The listing builds one solid part. Answer for the finished solid, in the listing's coordinates (mm). A direction names the side the tool comes from. Coordinates: 2 decimals unless noted, no trailing zeros. Loops run counter-clockwise (first coordinate to the right, second up) from the corner with the lowest first, then second, coordinate; pieces in that order, holes last. Notation, with made-up numbers: M 28,65.5 L 55,65.5 A27 ccw 55,87.5 Z; hole C 44,85 d8. An arc over 180 degrees is marked long. Answer as a JSON object with one key per item and string values. Group by question number.
1. A cutting plane is placed at B-B on z = -3. Give the vertices of the cut face in (x, y) (3 decimals).
2. A cutting plane is placed at C-C on x = -25.5. Give the vertices of the cut face in (y, z) (3 decimals).
3. A cutting plane is placed at A-A on y = -25.4. Give the vertices of the cut face in (x, z), and give its area (3 significant figures).
4. For faces 1 (the face through (-18.455, -42.037, -14.166)), 2 (the face through (-57.15, -20, -23)), determine the directions among +Z, -Z, +X, -X, +Y, -Y from which every point of the face is accessible in a straight line to the end or side of a thin tool.
5. Determine the mould class of faces 3 (the face through (-29, 0, -16)), 4 (the face through (-18.374, -8.961, -14.166)), 5 (the face through (-29, -25, -31.75)) for opening direction Y: released by +Y, released by -Y, zero draft, split by the parting line, or undercut.
6. Straight lines are drawn through the part: L1, parallel to Y at x = -40, z = -16; L2, parallel to Y at x = -27, z = -16; L3, parallel to Z at x = -25.5, y = -25.4. For each, find the intervals that lie inside material, in ascending order.
from build123d import *

# Parameters (mm, degrees)
F0_W     = 57.15
F0_H     = 50.8
F1_DEPTH = 31.75
F2_D     = 5.4102
F2_DEPTH = 27.94
F2_TIP   = 1.6253880605
F3_R     = 8.3312
F4_DEPTH = 57.151


with BuildPart() as f1:
    # F0 (on Top) → F1 (new body)
    with BuildSketch(Plane.XY):
        with Locations((-28.575, -25.4)):
            Rectangle(F0_W, F0_H)
    extrude(amount=-F1_DEPTH)

    # F2
    with Locations(Plane.XY):
        with Locations((-15.875, -7.9248), (-15.875, -42.8498), (-41.275, -42.8498), (-41.275, -7.9248)):
            Hole(F2_D / 2, depth=F2_DEPTH)
            with Locations((0, 0, -(F2_DEPTH + F2_TIP / 2))):  # 118° drill point
                Cone(0, F2_D / 2, F2_TIP, mode=Mode.SUBTRACT)

    # F3 (on face) → F4 (cut, through all)
    with BuildSketch(Plane.YZ):
        with Locations((-25.4, -15.875)):
            Circle(F3_R)
    extrude(amount=-F4_DEPTH, mode=Mode.SUBTRACT)


solid = f1.part
From the geometry:
{
 "1": {"outline": "M -57.15,-50.8 L 0,-50.8 L 0,0 L -57.15,0 Z; hole C -41.275,-42.85 d5.41; hole C -41.275,-7.925 d5.41; hole C -15.875,-42.85 d5.41; hole C -15.875,-7.925 d5.41"},
 "2": {"outline": "M -50.8,-31.75 L 0,-31.75 L 0,0 L -50.8,0 Z; hole C -25.4,-15.875 d16.662"},
 "3": {"outline": "M -57.15,-31.75 L 0,-31.75 L 0,-24.21 L -57.15,-24.21 Z; M -57.15,-7.54 L 0,-7.54 L 0,0 L -57.15,0 Z", "area": "862 mm²"},
 "4": {"face 1": "+Z", "face 2": "+Z, -Z, -X, +Y, -Y"},
 "5": {"face 3": "released by +Y", "face 4": "undercut", "face 5": "zero draft"},
 "6": {"L1": "y = -50.8 to -45.24, -40.46 to -33.73, -17.07 to -10.31, -5.54 to 0", "L2": "y = -50.8 to -33.73, -17.07 to 0", "L3": "z = -31.75 to -24.21, -7.54 to 0"}
}
